CAD build for the part. Positions are in the model's coordinates, mm. Coordinates: 2 decimals unless noted, no trailing zeros. Loops run counter-clockwise (first coordinate to the right, second up) from the corner with the lowest first, then second, coordinate; pieces in that order, holes last. Notation, with made-up numbers: (-30, 46.25) -> (19, 46.25) arc R10 cw to (19, 59.25) -> close; hole circle Ø8 at (16.5, -35.75). An arc over 180 degrees is marked (long way). Return JSON: item names as keys, results as strings. Group by question number.
(1) Saw through at A-A on z = 65. Write the cut outline in (x, y), then the cut area to 3 significant figures.
(2) Flat gauge pins, fed straight in: pin 1 Ø2 at (x, z) = (-48.5, 32.5) entering from +Y; pin 2 Ø1.7 at (y, z) = (13.5, 42) entering from +X; pin 3 Ø1.1 at (x, y) = (60, 12) entering from -Z. Where does each tip first touch, or does it go through?
(3) Saw through at B-B on x = -38.5. Write the cut outline in (y, z), then the cut area to 3 significant figures.
(4) Probe L1, parallel to Z at x = -47, y = 13.25; L2, parallel to Z at x = 16.5, y = 11.4; L3, parallel to X at y = 12.65, z = 97.5. List the from-to ranges inside material, lowest first.
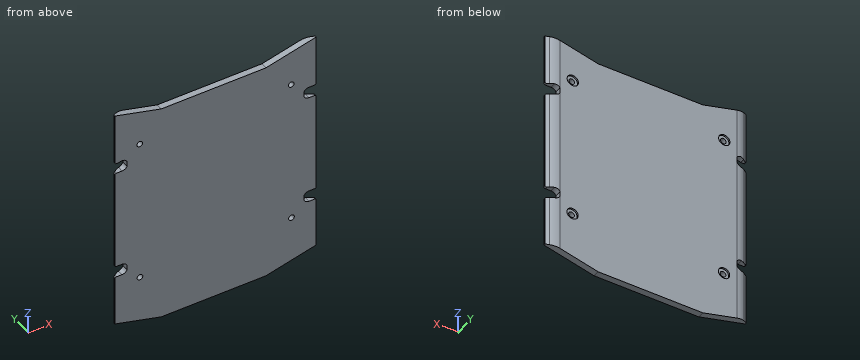
```python
from build123d import *

# Parameters (mm, degrees)
BOSS_EXTRUDE1_DEPTH    = 148
FILLET1_R              = 10
CUT_EXTRUDE1_DEPTH     = 10
CUT_EXTRUDE2_START     = -4
CUT_EXTRUDE2_OUTLINE_R = 1.75
CUT_EXTRUDE2_DEPTH     = 4
SKETCH4_R              = 3.5
CUT_EXTRUDE3_DEPTH     = 1
FILLET2_R              = 1


# Read off the part's stored shape, not the designer's step: Cut-Extrude2
with BuildPart() as part:
    # Sketch1 → Boss-Extrude1 (new body)
    with BuildSketch(Plane.XY):
        Polygon((57.875, 15), (-57.875, 15), (-62.5, 12), (-62.5, 11), (62.5, 11), (62.5, 12), align=None)
    extrude(amount=BOSS_EXTRUDE1_DEPTH)

    # Fillet1
    fillet1_edges = [part.edges().sort_by_distance(p)[0] for p in [
        (-57.875, 15, 74),
        (57.875, 15, 74),
    ]]
    fillet(fillet1_edges, radius=FILLET1_R)

    # Sketch2 → Cut-Extrude1 (cut)
    with BuildSketch(Plane(origin=(0, 15, 0), x_dir=(1, 0, 0), z_dir=(0, 1, 0))):
        Polygon((-62.5, -7.5), (-33.66084425, 0), (31.256498232, 0), (62.5, -7.5), (62.5, 0), (31.256498232, 7.5), (-33.66084425, 7.5), (-62.5, 0), align=None)
        Polygon((31.256498232, -148), (62.5, -155.5), (62.5, -148), (31.256498232, -140.5), (-33.66084425, -140.5), (-62.5, -148), (-62.5, -155.5), (-33.66084425, -148), align=None)
    extrude(amount=-CUT_EXTRUDE1_DEPTH, mode=Mode.SUBTRACT)

    # Cut-Extrude2 outline → Cut-Extrude2 (cut)
    with BuildSketch(Plane(origin=(0, 15, 0), x_dir=(1, 0, 0), z_dir=(0, 1, 0)).offset(CUT_EXTRUDE2_START)):
        with BuildLine():
            Line((-62.5, -38.943696852), (-62.5, -45.943696852))
            Line((-62.5, -45.943696852), (-57.999999085, -45.943696852))
            ThreePointArc((-57.999999085, -45.943696852), (-56.202906175, -45.447104429), (-54.915769107, -44.098243751))
            Line((-54.915769107, -44.098243751), (-54.915769107, -40.789149953))
            ThreePointArc((-54.915769107, -40.789149953), (-56.202906175, -39.440289275), (-57.999999085, -38.943696852))
            Line((-57.999999085, -38.943696852), (-62.5, -38.943696852))
        make_face()
        with BuildLine():
            Line((-62.5, -115.432850877), (-59.820701756, -115.432850877))
            ThreePointArc((-59.820701756, -115.432850877), (-57.081076151, -115.820911776), (-54.915769107, -114.098243751))
            Line((-54.915769107, -114.098243751), (-54.915769107, -110.789149953))
            ThreePointArc((-54.915769107, -110.789149953), (-56.202906175, -109.440289275), (-57.999999085, -108.943696852))
            Line((-57.999999085, -108.943696852), (-62.5, -108.943696852))
            Line((-62.5, -108.943696852), (-62.5, -115.432850877))
        make_face()
        with BuildLine():
            Line((57.999999085, -45.943696852), (62.5, -45.943696852))
            Line((62.5, -45.943696852), (62.5, -38.943696852))
            Line((62.5, -38.943696852), (57.999999085, -38.943696852))
            ThreePointArc((57.999999085, -38.943696852), (56.202906175, -39.440289275), (54.915769107, -40.789149953))
            Line((54.915769107, -40.789149953), (54.915769107, -44.098243751))
            ThreePointArc((54.915769107, -44.098243751), (56.202906175, -45.447104429), (57.999999085, -45.943696852))
        make_face()
        with BuildLine():
            Line((62.5, -108.943696852), (57.999999085, -108.943696852))
            ThreePointArc((57.999999085, -108.943696852), (56.202906175, -109.440289275), (54.915769107, -110.789149953))
            Line((54.915769107, -110.789149953), (54.915769107, -114.098243751))
            ThreePointArc((54.915769107, -114.098243751), (56.202906175, -115.447104429), (57.999999085, -115.943696852))
            Line((57.999999085, -115.943696852), (62.5, -115.943696852))
            Line((62.5, -115.943696852), (62.5, -108.943696852))
        make_face()
        with Locations((47.15, -32.480990458)):
            Circle(CUT_EXTRUDE2_OUTLINE_R)
        with Locations((-47, -122.447604366)):
            Circle(CUT_EXTRUDE2_OUTLINE_R)
        with Locations((46.999994071, -122.480990458)):
            Circle(CUT_EXTRUDE2_OUTLINE_R)
        with Locations((-46.85, -32.447604366)):
            Circle(CUT_EXTRUDE2_OUTLINE_R)
    extrude(amount=CUT_EXTRUDE2_DEPTH, mode=Mode.SUBTRACT)

    # Sketch4 → Cut-Extrude3 (cut)
    with BuildSketch(Plane(origin=(0, 15, 0), x_dir=(1, 0, 0), z_dir=(0, 1, 0))):
        with Locations(Location((-46.85, -32.447604366, 0), (0, 0, 270))):
            Circle(SKETCH4_R)
        with Locations(Location((47.15, -32.480990458, 0), (0, 0, 270))):
            Circle(SKETCH4_R)
        with Locations(Location((-47, -122.447604366, 0), (0, 0, 270))):
            Circle(SKETCH4_R)
        with Locations(Location((46.999994071, -122.480990458, 0), (0, 0, 270))):
            Circle(SKETCH4_R)
    extrude(amount=-CUT_EXTRUDE3_DEPTH, mode=Mode.SUBTRACT)

    # Fillet2
    fillet2_edges = [part.edges().sort_by_distance(p)[0] for p in [
        (62.5, 11.5, 115.943696852),
        (62.5, 11.5, 108.943696852),
        (-62.5, 11.5, 45.943696852),
        (-62.5, 11.5, 38.943696852),
        (-62.5, 11.5, 115.432850877),
        (-62.5, 11.5, 108.943696852),
        (62.5, 11.5, 45.943696852),
        (62.5, 11.5, 38.943696852),
    ]]
    fillet(fillet2_edges, radius=FILLET2_R)


solid = part.part
```
Geometry results:
{
 "1": {"outline": "(-62.5, 11) -> (62.5, 11) -> (62.5, 12) -> (60.36, 13.39) arc R10 ccw to (54.92, 15) -> (-54.92, 15) arc R10 ccw to (-60.36, 13.39) -> (-62.5, 12) -> close", "area": "484 mm²"},
 "2": {"pin 1": "y = 14", "pin 2": "x = 54.92", "pin 3": "z = 6.77"},
 "3": {"outline": "(11, 1.26) -> (15, 1.26) -> (15, 141.76) -> (11, 141.76) -> close", "area": "562 mm²"},
 "4": {"L1": "3.47 to 30.7, 34.19 to 120.7, 124.2 to 143.97", "L2": "0 to 140.5", "L3": "-61.5 to 61.5"}
}
